from build123d import *

# Parameters (mm, degrees)
REVOLVE3_ANGLE = 359


with BuildPart() as part:
    # Sketch1 → Revolve3 (revolve)
    with BuildSketch(Plane.XY):
        with BuildLine():
            Line((25.4, 0), (0, 25.4))
            Line((0, 25.4), (0, 114.740562784))
            Line((0, 114.740562784), (33.369066404, 50.8))
            Line((33.369066404, 50.8), (58.29289998, 50.8))
            Line((58.29289998, 50.8), (67.24644999, 41.84644999))
            Line((67.24644999, 41.84644999), (76.2, 50.8))
            Line((76.2, 50.8), (104.441096188, 50.8))
            ThreePointArc((104.441096188, 50.8), (120.39265005, 44.19265005), (127, 28.241096188))
            Line((127, 28.241096188), (127, 0))
            Line((127, 0), (25.4, 0))
        make_face()
    revolve(axis=Axis((0, 25.4, 0), (0, -1, 0)), revolution_arc=REVOLVE3_ANGLE)


solid = part.part
Part model, mm, in its own coordinate system. A direction names the side the tool comes from. Give positions to 0.01 mm unless a question says otherwise; leave off trailing zeros. Loops run counter-clockwise (first coordinate to the right, second up) from the corner with the lowest first, then second, coordinate; pieces in that order, holes last. Notation, with made-up numbers: (35.5, 5) -> (54.5, 5) arc R34 ccw to (54.5, 41) -> close; hole circle Ø3 at (42.25, 50). An arc over 180 degrees is marked (long way). Write each question's results on one line, items separated by ' | '. Start each with the question number.
Q1. Wall check: L1, parallel to Y at x = 34.5, z = 38; L2, parallel to Z at x = 116.5, y = 15.5; L3, parallel to Z at x = 20.5, y = 66.5. Give the ranges that are in metal, low to high.
Q2. Pin check, flat tips, straight feed: P1, Ø10, axis at x = -5, y = 43, coming from the +Z side; P2, Ø5, axis at x = -99.5, z = -59.5, coming from the +Y side; P3, Ø12, axis at y = 32, z = 61.5, coming from the +X side. Stop position of each tip, or through.
Q3. Band-saw the part on B-B on y = 31.5. List the corners of the cut face in (x, z).
Q4. Pull direction Z, two halves, no side cores. Call faces 3 (the face through (50, 33, 0)), 4 (the face through (-13.19, 89.43, 0.69)), 5 (the face through (-25, 50.8, -25)): +Z half, -Z half, draft (parallel to the pull), parting line (faces both ways), or undercut.
Q5. Band-saw the part on A-A on y = 82. List the corners of the cut face in (x, z), plus the area to 3 significant figures.
Q6. Which spindle directions (+Z, -Z, +X, -X, +Y, -Y) get a long thin tool onto all of the face, cutting with end or side? Do faces 1 (the face through (-7, 50.8, -77)), 2 (the face through (-6.87, 18.52, 0.36)). Say none if no direction does.
Results are:
1) L1: y = 0 to 50.8 | L2: z = -50.56 to -2.03, 0 to 50.56 | L3: z = -14.61 to -0.36, 0 to 14.61
2) P1: stops at z = 124.69 | P2: stops at y = 48.93 | P3: stops at x = 114.01
3) outline: (0, 0) -> (126.76, 0) arc R126.76 ccw (long way) to (126.74, -2.21) -> close
4) face 3: undercut | face 4: parting line | face 5: draft
5) outline: (0, 0) -> (17.09, 0) arc R17.09 ccw (long way) to (17.08, -0.3) -> close | area: 915 mm²
6) face 1: +Y | face 2: -Y
